Geometry check sheet. Reference: the model listing, model coordinates, mm. Face numbers are marked on the shaded views. A direction names the side the tool comes from. Coordinates: 2 decimals unless noted, no trailing zeros. Loops run counter-clockwise (first coordinate to the right, second up) from the corner with the lowest first, then second, coordinate; pieces in that order, holes last.
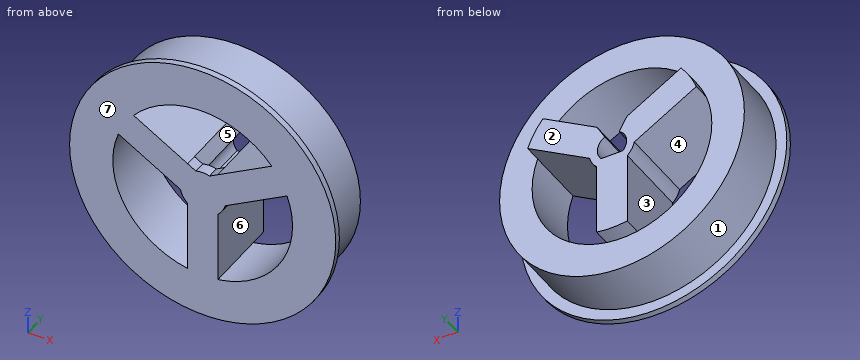
Autodesk Inventor part; units mm, degrees
ref_plane "YZ Plane" through (0, 0, 0) normal (1, 0, 0) x (0, 1, 0)
ref_plane "XZ Plane" through (0, 0, 0) normal (0, 1, 0) x (-1, 0, 0)
ref_plane "XY Plane" through (0, 0, 0) normal (0, 0, 1) x (1, 0, 0)
sketch "Sketch1" plane through (0, 0, 0) normal (0, 1, 0) x (-1, 0, 0)
  circle A0 centre (0, 0) radius 11.75
  dimension "d0" = 23.5
extrude "Extrusion1" add sketch "Sketch1" along normal blind 2.2
sketch "Sketch2" plane through (0, 0, 0) normal (0, -1, 0) x (1, 0, 0)
  circle A0 centre (0, 0) radius 16
  dimension "d3" = 32
extrude "Extrusion2" add sketch "Sketch2" along normal blind 7
sketch "Sketch3" plane through (0, 2.2, 0) normal (0, 1, 0) x (1, 0, 0)
  arc A0 (-1.425, 1.2718) -> (1.425, 1.2718) centre (0, 0) ccw
  line L0 (-1.425, 1.2718) -> (1.425, 1.2718)
  dimension "d6" = 3.82
  dimension "d7" = 2.85
extrude "Extrusion3" cut sketch "Sketch3" against normal blind 8.5
sketch "Sketch6" plane through (0, -7, 0) normal (0, -1, 0) x (1, 0, 0)
  circle A0 centre (0, 0) radius 17.4
  circle A1 centre (0, 0) radius 16
  dimension "d16" = 1.4
extrude "Extrusion6" add sketch "Sketch6" along normal blind 0.8 contours A0 | A1
sketch "Sketch7" plane through (0, 2.2, 0) normal (0, 1, 0) x (1, 0, 0)
  circle A0 centre (0, 0) radius 11.75
  line L0 (-1.425, 1.2718) -> (1.425, 1.2718)
  arc A1 (-1.425, 1.2718) -> (1.425, 1.2718) centre (0, 0) ccw
  circle A2 centre (0, 0) radius 11.75
  line L1 (-2, 11.5785) -> (-2, 2.1889)
  line L2 (2, 2.1889) -> (2, 11.5785)
  line L3 (1.8733, 0.3725) -> (1.9126, 0.3725)
  line L4 (0, 0) -> (0, 15.765) construction
  line L5 (-2.8956, 0.6376) -> (-11.0273, -4.0572)
  line L6 (-9.0273, -7.5213) -> (-0.8956, -2.8265)
  line L7 (0.8956, -2.8265) -> (9.0273, -7.5213)
  line L8 (11.0273, -4.0572) -> (2.8956, 0.6376)
  line L9 (-1.525, 1.2942) -> (-1.525, 15.9272)
  arc A3 (11.0273, -4.0572) -> (2, 11.5785) centre (0, 0) ccw
  arc A4 (-2, 11.5785) -> (-11.0273, -4.0572) centre (0, 0) ccw
  arc A5 (-9.0273, -7.5213) -> (9.0273, -7.5213) centre (0, 0) ccw
  arc A6 (2.8956, 0.6376) -> (2, 2.1889) centre (0, 0) ccw
  arc A7 (-1.425, 1.2718) -> (1.425, 1.2718) centre (0, 0) ccw
  line L10 (1.965, -3.4439) -> (0, 0)
  line L11 (0, 0) -> (-1.965, -3.4439)
  arc A8 (1.4757, -2.5863) -> (-1.525, -2.5576) centre (0, 0) ccw
  arc A9 (-2, 2.1889) -> (-2.8956, 0.6376) centre (0, 0) ccw
  arc A10 (2.8956, 0.6376) -> (2, 2.1889) centre (0, 0) ccw
  arc A11 (1.4757, -2.5863) -> (-1.525, -2.5576) centre (0, 0) ccw
  dimension "d20" = 4
  dimension "d23" = 360
extrude "Extrusion7" cut sketch "Sketch7" against normal blind 10 contours A0 L8 A8 L2 | A0 L6 L11 A1 L10 L7 | L1 A8 L5 A0 | A1 L11 L10
sketch "Sketch8" plane through (0, -7.8, 0) normal (0, -1, 0) x (1, 0, 0)
  arc A0 (2, -2.1889) -> (2.8956, -0.6376) centre (0, 0) ccw
  line L0 (0, 0) -> (-1.965, 3.4439)
  line L1 (-1.965, 3.4439) -> (-9.0273, 7.5213)
  line L2 (-1.965, 3.4439) -> (-0.8956, 2.8265)
  line L3 (0.8956, 2.8265) -> (1.965, 3.4439)
  line L4 (0.9466, 1.659) -> (1.965, 3.4439)
  line L5 (1.965, 3.4439) -> (1.4558, 2.5514)
  line L6 (-1.965, 3.4439) -> (-1.4694, 2.5753)
  arc A1 (-1.4694, 2.5753) -> (1.4694, 2.5753) centre (0, 0) ccw
  arc A2 (0.8956, 2.8265) -> (-0.8956, 2.8265) centre (0, 0) ccw
extrude "Extrusion8" add sketch "Sketch8" against normal blind 1.5
properties part number "wheelPixi1"
(1) Access from +Z, -Z, +X, -X, +Y, -Y to the whole of each face (thin tool, end or side, straight path). Record for the marked faces 5, 6 and 7.
Findings:
face 5: +Y
face 6: +Y, -Y
face 7: +Z, -Z, +X, -X, -Y
(2) Sectioned sample at A-A on x = 0. Record the cut outline in (y, z) (3 decimals).
Findings:
outline: (-7.8, -17.4) - (-7, -17.4) - (-7, -16) - (0, -16) - (0, -11.75) - (2.2, -11.75) - (2.2, -1.272) - (-6.3, -1.272) - (-6.3, 2.965) - (-7.8, 2.965) - close; (-7.8, 11.75) - (0, 11.75) - (0, 16) - (-7, 16) - (-7, 17.4) - (-7.8, 17.4) - close
(3) Gauge pin test, flat ends, axial feed: pin 1 Ø1 at (x, y) = (2, -2) entering from +Z; pin 2 Ø2 at (y, z) = (-4.5, 13) entering from -X; pin 3 Ø3 at (x, y) = (-0.5, -1.5) entering from +Z. Record the tip position at first contact, or that the pin passes through.
Findings:
pin 1: stops at z = 15.93
pin 2: stops at x = -10.58
pin 3: stops at z = 16
(4) Sectioned sample at B-B on z = 8.5. Record the cut outline in (x, y).
Findings:
outline: (-15.18, -7.8) - (-8.11, -7.8) - (-8.11, 0) - (-13.56, 0) - (-13.56, -7) - (-15.18, -7) - close; (8.11, -7.8) - (15.18, -7.8) - (15.18, -7) - (13.56, -7) - (13.56, 0) - (8.11, 0) - close
(5) Sectioned sample at C-C on y = -2.5. State how many separate pieces and enclosed holes the cut face has, and give its area (3 significant figures).
Findings:
separate pieces: 1
enclosed holes: 3
area: 492 mm2
(6) Sectioned sample at D-D on x = 4. Record the cut outline in (y, z).
Findings:
outline: (-7.8, -16.93) - (-7, -16.93) - (-7, -15.49) - (0, -15.49) - (0, -11.05) - (-7.8, -11.05) - close; (-7.8, 0) - (2.2, 0) - (2.2, 4.62) - (-7.8, 4.62) - close; (-7.8, 11.05) - (0, 11.05) - (0, 15.49) - (-7, 15.49) - (-7, 16.93) - (-7.8, 16.93) - close
(7) Scan lines: L1, parallel to Z at x = 6.5, y = -5.5; L2, parallel to X at y = -7.5, z = -1; L3, parallel to X at y = -3.5, z = -0.5. Record each from-to range of solid material in increasing order.
Findings:
L1: z = -14.62 to -9.79, 1.44 to 6.06, 9.79 to 14.62
L2: x = -17.37 to -11.71, -2.8 to 2.8, 11.71 to 17.37
L3: x = -15.99 to -11.74, -3.13 to -1.84, 1.84 to 3.13, 11.74 to 15.99
(8) Draft check along X on the marked faces 1, 2, 3 and 4. Enter one of: +X half, -X half, draft (parallel to the pull), parting line (faces both ways), or undercut.
Findings:
face 1: parting line
face 2: draft
face 3: undercut
face 4: undercut
